Here's the drawing with two shaded views (mm, measured from the low corner). I have some questions. Coordinates: 2 decimals unless noted, no trailing zeros. Write each loop counter-clockwise with the first axis right and the second up, starting at its lowest first coordinate (ties: lowest second). Pieces come first, ordered by that corner, then holes. Notation, with made-up numbers: (-24.5, 80.25) - (-10.5, 80.25) arc R10 cw to (-10.5, 85.25) - close; hole circle Ø2 at (47.25, 86.5). An arc over 180 degrees is marked (long way). Answer in a Markdown table with one row per item. Add a question column.
Item 1: Imagine slicing it at B-B (y = 29). Please give me the cut outline in (x, z).
Item 2: If I drill on probe 1 along Y at (x, z) = (18.5, 2.7); probe 2 along X at (y, z) = (70, 1.9); probe 3 along Y at (x, z) = (61.5, 0.95), over which ranges is the centre line in solid material (lowest first)? Write a range as from..to.
Item 3: Imagine slicing it at C-C (z = 2.4). Please give me the cut outline in (x, y), plus the area to 3 significant figures.
Item 4: Imagine slicing it at A-A (x = 48). Please give me the cut outline in (y, z), plus the area to 3 significant figures.
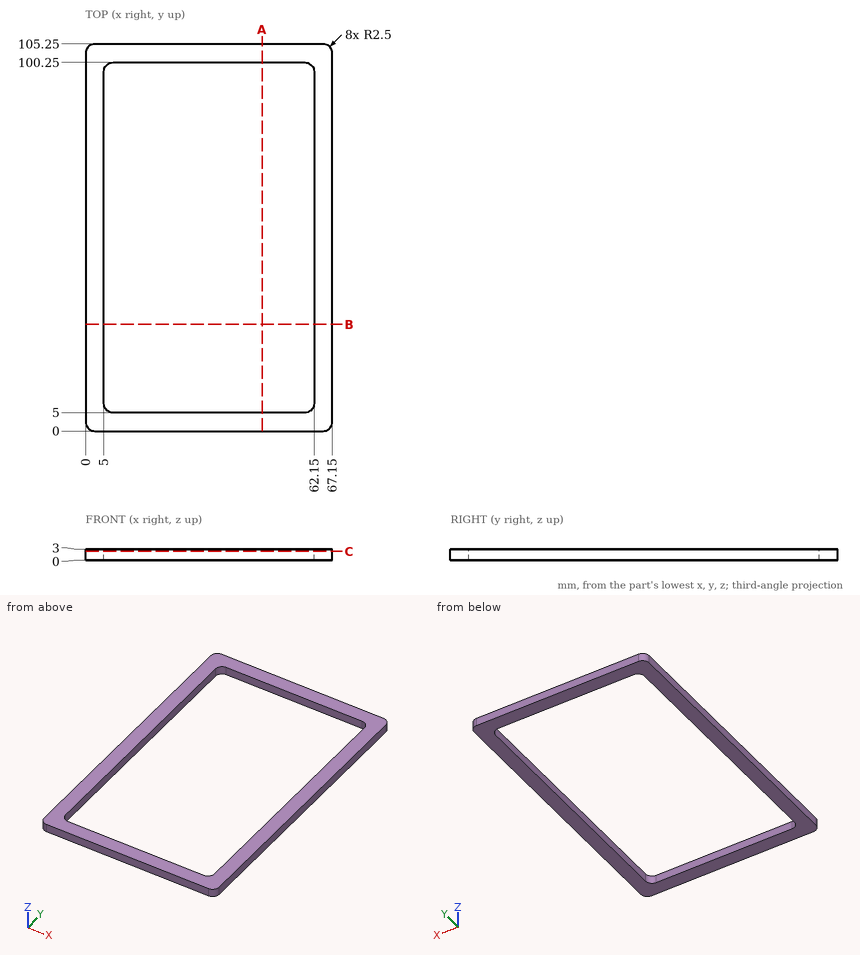
Here are the results:
| question | item | result |
|---|---|---|
| 1 | outline | (0, 0) - (5, 0) - (5, 3) - (0, 3) - close; (62.15, 0) - (67.15, 0) - (67.15, 3) - (62.15, 3) - close |
| 2 | probe 1 | y = 0..5, 100.25..105.25 |
| 2 | probe 2 | x = 0..5, 62.15..67.15 |
| 2 | probe 3 | y = 0..5.82, 99.43..105.25 |
| 3 | outline | (0, 2.5) arc R2.5 ccw to (2.5, 0) - (64.65, 0) arc R2.5 ccw to (67.15, 2.5) - (67.15, 102.75) arc R2.5 ccw to (64.65, 105.25) - (2.5, 105.25) arc R2.5 ccw to (0, 102.75) - close; hole (5, 7.5) arc R2.5 ccw to (7.5, 5) - (59.65, 5) arc R2.5 ccw to (62.15, 7.5) - (62.15, 97.75) arc R2.5 ccw to (59.65, 100.25) - (7.5, 100.25) arc R2.5 ccw to (5, 97.75) - close |
| 3 | area | 1,620 mm2 |
| 4 | outline | (0, 0) - (5, 0) - (5, 3) - (0, 3) - close; (100.25, 0) - (105.25, 0) - (105.25, 3) - (100.25, 3) - close |
| 4 | area | 30.0 mm2 |
